Source: three-view drawing plus pictorial views. Frame: mm from the lowest corner of the part. A direction names the side the tool comes from. Round coordinates to 2 decimals unless told otherwise and drop trailing zeros. Order: outer loops, then holes, each group sorted by start corner. A loop starts at its lowest first (then second) coordinate and runs counter-clockwise, first axis right, second up. Notation, with made-up numbers: (23, 32) - (52, 32) arc R21 ccw to (52, 50) - close; hole circle Ø7 at (76, 83). An arc over 180 degrees is marked (long way). Use one line per item in the form item = value. Start each with the question number.
Q1. Draft query along Z for the marked faces 1, 2 and 3. Return one class per face: released by +Z, released by -Z, zero draft, split by the parting line, or undercut.
Q2. Pin query (flat end, axial travel): pin 1 Ø10 at (x, y) = (54, 16.5) entering from +Z; pin 2 Ø13 at (x, z) = (48.89, 24.3) entering from +Y; pin 3 Ø3 at (x, y) = (30, 15) entering from -Z; pin 4 Ø3 at (x, z) = (41.5, 49.5) entering from -Y. Return the tip coordinate at first contact, or that it passes through.
Q3. Set-up query: the marked faces 4 and 5. Return all of +Z, -Z, +X, -X, +Y, -Y with unobstructed straight access to the full face (end or side cutting, diameter ignored); none if empty.
Q4. Ray query, line 1 (Z direction, x = 52.5, y = 21.75) (1 decimal); line 2 (Y direction, x = 61, z = 36.5); line 3 (Z direction, x = 31.5, y = 23). Return the intervals inside material, ascending. Write a range as [from, to].
Q5. Cut plane B-B, the plane z = 33.3. Return the cut outline in (x, y), and give its area (3 significant figures).
Q6. Cut plane A-A, the plane x = 33.3. Return the cut outline in (y, z) (1 decimal).
Q7. Cut plane D-D, the plane y = 13.5. Give the number of separate pieces and of enclosed holes in the cut face, and give its area (3 significant figures).
Q8. Cut plane C-C, the plane z = 49. Return the cut outline in (x, y).
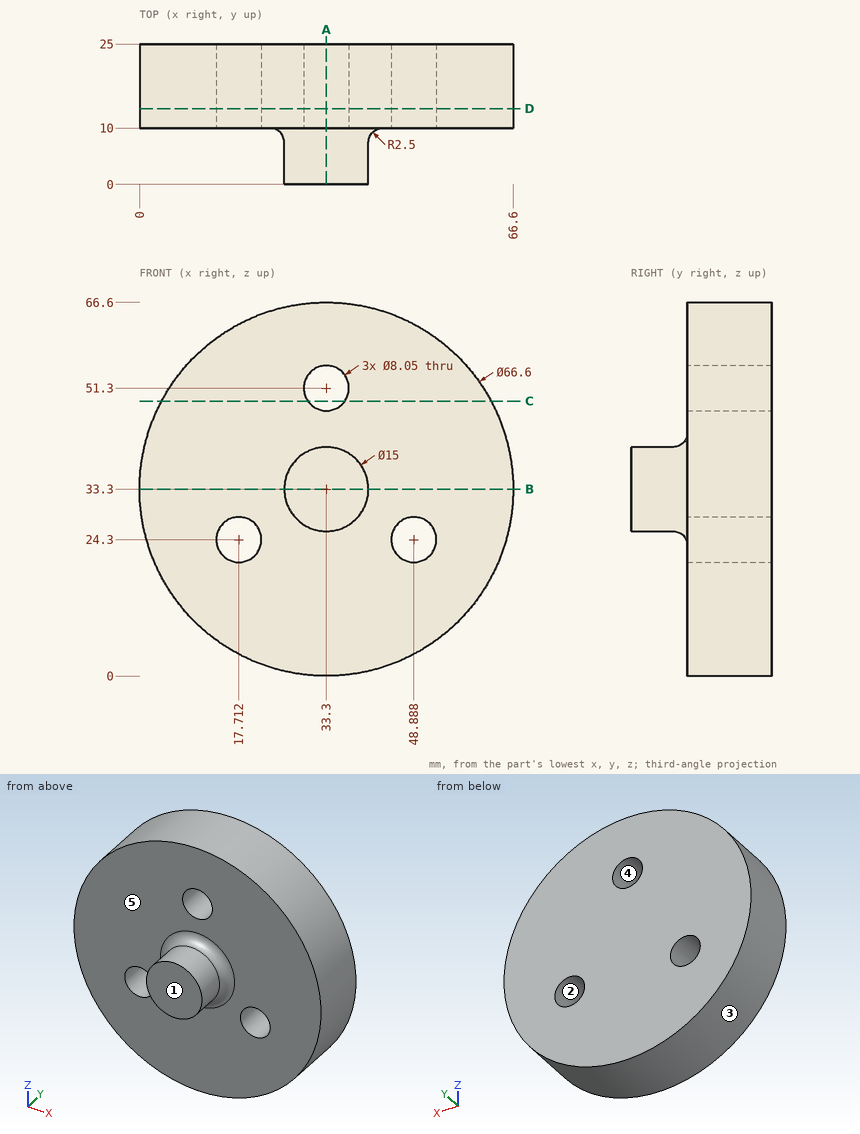
Completed:
q1.face_1 = zero draft
q1.face_2 = undercut
q1.face_3 = split by the parting line
q2.pin_1 = 62.67
q2.pin_2 = 25
q2.pin_3 = 0.05
q2.pin_4 = 10
q3.face_4 = +Y, -Y
q3.face_5 = -Y
q4.line_1 = [6.1, 22.5], [26.1, 60.5]
q4.line_2 = [10, 25]
q4.line_3 = [0.05, 47.7], [54.9, 66.55]
q5.outline = (0, 10) - (23.3, 10) arc R2.5 cw to (25.8, 7.5) - (25.8, 0) - (40.8, 0) - (40.8, 7.5) arc R2.5 cw to (43.3, 10) - (66.6, 10) - (66.6, 25) - (0, 25) - close
q5.area = 1,150 mm2
q6.outline = (0, 25.8) - (7.5, 25.8) arc R2.5 cw to (10, 23.3) - (10, 0) - (25, 0) - (25, 47.3) - (10, 47.3) - (10, 43.3) arc R2.5 cw to (7.5, 40.8) - (0, 40.8) - close; (10, 55.3) - (25, 55.3) - (25, 66.6) - (10, 66.6) - close
q7.separate_pieces = 1
q7.enclosed_holes = 3
q7.area = 3,330 mm2
q8.outline = (3.93, 10) - (30, 10) - (30, 25) - (3.93, 25) - close; (36.6, 10) - (62.67, 10) - (62.67, 25) - (36.6, 25) - close
